The listing builds one solid part. Answer for the finished solid, in the listing's coordinates (mm). A direction names the side the tool comes from. Coordinates: 2 decimals unless noted, no trailing zeros. Write each loop counter-clockwise with the first axis right and the second up, starting at its lowest first coordinate (ties: lowest second). Pieces come first, ordered by that corner, then holes.
from build123d import *

# Parameters (mm, degrees)
BOSS_EXTRU_1_DEPTH        = 13
COQUE1_T                  = -5
COQUE1_THICKNESS_2_FACE_W = 65
COQUE1_THICKNESS_2_FACE_H = 65
COQUE1_THICKNESS_2_DEPTH  = 2
ENL_V_MAT_EXTRU_1_REACH   = 88.587
ESQUISSE2_R               = 2.5
ENL_V_MAT_EXTRU_2_REACH   = 95.396
ESQUISSE3_R               = 2.5
ESQUISSE4_W               = 18
ESQUISSE4_H               = 18
ESQUISSE4_W_2             = 15
ESQUISSE4_H_2             = 15
BOSS_EXTRU_2_DEPTH        = 10
ESQUISSE5_R               = 11.5
ESQUISSE5_R_2             = 14.5
ENL_V_MAT_EXTRU_3_DEPTH   = 13


with BuildPart() as part:
    # Esquisse1 → Boss.-Extru.1 (new body)
    with BuildSketch(Plane.XY):
        Polygon((44.118436308, 33.728448276), (54.118436308, 33.728448276), (54.118436308, 23.728448276), (54.118436308, -41.271551724), (-20.881563692, -41.271551724), (-20.881563692, 33.728448276), align=None)
    extrude(amount=BOSS_EXTRU_1_DEPTH)

    # Coque1
    coque1_openings = [part.faces().sort_by_distance(p)[0] for p in [
        (16.618436308, -3.771551724, 13),
    ]]
    offset(amount=COQUE1_T, openings=coque1_openings, kind=Kind.INTERSECTION)

    # Coque1 thickness 2 face (on inner face of the shell) → Coque1 thickness 2 (cut)
    with BuildSketch(Plane(origin=(16.618436308, -3.771551724, 5), x_dir=(-1, 0, 0), z_dir=(0, 0, -1))):
        Rectangle(COQUE1_THICKNESS_2_FACE_W, COQUE1_THICKNESS_2_FACE_H)
    extrude(amount=COQUE1_THICKNESS_2_DEPTH, mode=Mode.SUBTRACT)

    # Enlèv. mat.-Extru.1: up to this face of the body (flat: up to its plane)
    enl_v_mat_extru_1_end = Plane(part.part.faces().sort_by_distance((54.118436308, -3.771551724, 6.5))[0])
    # Esquisse2 → Enlèv. mat.-Extru.1 (cut, up to the picked face)
    with BuildSketch(Plane.ZY.offset(20.881563692), mode=Mode.PRIVATE) as enl_v_mat_extru_1_sk1:
        with Locations(Location((8, -16.271551724, 0), (0, 0, 270))):
            Circle(ESQUISSE2_R)
    enl_v_mat_extru_1_tool1 = split(extrude(enl_v_mat_extru_1_sk1.sketch, amount=-ENL_V_MAT_EXTRU_1_REACH, mode=Mode.PRIVATE), bisect_by=enl_v_mat_extru_1_end, keep=Keep.BOTH, mode=Mode.PRIVATE)
    # Esquisse2 → Enlèv. mat.-Extru.1 (cut, up to the picked face)
    with BuildSketch(Plane.ZY.offset(20.881563692), mode=Mode.PRIVATE) as enl_v_mat_extru_1_sk2:
        with Locations(Location((8, 8.728448276, 0), (0, 0, 270))):
            Circle(ESQUISSE2_R)
    enl_v_mat_extru_1_tool2 = split(extrude(enl_v_mat_extru_1_sk2.sketch, amount=-ENL_V_MAT_EXTRU_1_REACH, mode=Mode.PRIVATE), bisect_by=enl_v_mat_extru_1_end, keep=Keep.BOTH, mode=Mode.PRIVATE)
    add(enl_v_mat_extru_1_tool1.solids().sort_by(Axis((-20.881564, -16.271552, 8), (1, 0, 0)))[0], mode=Mode.SUBTRACT)
    add(enl_v_mat_extru_1_tool2.solids().sort_by(Axis((-20.881564, 8.728448, 8), (1, 0, 0)))[0], mode=Mode.SUBTRACT)

    # Enlèv. mat.-Extru.2: up to this face of the body (flat: up to its plane)
    enl_v_mat_extru_2_end = Plane(part.part.faces().sort_by_distance((16.618436308, 33.728448276, 6.5))[0])
    # Esquisse3 → Enlèv. mat.-Extru.2 (cut, up to the picked face)
    with BuildSketch(Plane.XZ.offset(41.271551724), mode=Mode.PRIVATE) as enl_v_mat_extru_2_sk1:
        with Locations(Location((4.118436308, 8, 0), (0, 0, 270))):
            Circle(ESQUISSE3_R)
    enl_v_mat_extru_2_tool1 = split(extrude(enl_v_mat_extru_2_sk1.sketch, amount=-ENL_V_MAT_EXTRU_2_REACH, mode=Mode.PRIVATE), bisect_by=enl_v_mat_extru_2_end, keep=Keep.BOTH, mode=Mode.PRIVATE)
    # Esquisse3 → Enlèv. mat.-Extru.2 (cut, up to the picked face)
    with BuildSketch(Plane.XZ.offset(41.271551724), mode=Mode.PRIVATE) as enl_v_mat_extru_2_sk2:
        with Locations(Location((29.118436308, 8, 0), (0, 0, 270))):
            Circle(ESQUISSE3_R)
    enl_v_mat_extru_2_tool2 = split(extrude(enl_v_mat_extru_2_sk2.sketch, amount=-ENL_V_MAT_EXTRU_2_REACH, mode=Mode.PRIVATE), bisect_by=enl_v_mat_extru_2_end, keep=Keep.BOTH, mode=Mode.PRIVATE)
    add(enl_v_mat_extru_2_tool1.solids().sort_by(Axis((4.118436, -41.271552, 8), (0, 1, 0)))[0], mode=Mode.SUBTRACT)
    add(enl_v_mat_extru_2_tool2.solids().sort_by(Axis((29.118436, -41.271552, 8), (0, 1, 0)))[0], mode=Mode.SUBTRACT)

    # Esquisse4 → Boss.-Extru.2 (add)
    with BuildSketch(Plane.XY.offset(3)):
        Polygon((-5.881563692, 28.728448276), (-15.881563692, 18.728448276), (-15.881563692, 28.728448276), align=None)
        Polygon((49.118436308, 28.728448276), (49.118436308, 18.728448276), (39.118436308, 28.728448276), align=None)
        with Locations((45.118436308, -32.271551724)):
            Rectangle(ESQUISSE4_W, ESQUISSE4_H)
        with Locations((-13.381563692, -33.771551724)):
            Rectangle(ESQUISSE4_W_2, ESQUISSE4_H_2)
    extrude(amount=BOSS_EXTRU_2_DEPTH)

    # Esquisse5 → Enlèv. mat.-Extru.3 (cut)
    with BuildSketch(Plane.XY.offset(13)):
        with Locations((-20.881563692, -41.271551724)):
            Circle(ESQUISSE5_R)
        with Locations((54.118436308, -41.271551724)):
            Circle(ESQUISSE5_R_2)
    extrude(amount=-ENL_V_MAT_EXTRU_3_DEPTH, mode=Mode.SUBTRACT)


solid = part.part
Q1. The part is cut by section B-B, the plane z = 8. State how many separate pieces and enclosed holes the cut face has, then the cut area to 3 significant figures.
Answers below:
separate pieces: 8
enclosed holes: 0
area: 1,300 mm2
Q2. The part is cut by section A-A, the plane y = -12.5. Write down the section's boundary in (x, z).
Answers below:
outline: (-20.88, 0) - (54.12, 0) - (54.12, 13) - (49.12, 13) - (49.12, 3) - (-15.88, 3) - (-15.88, 13) - (-20.88, 13) - close
Q3. Find the intervals of material crossed by probe 1 along X at (y, z) = (12.5, 4.5); probe 2 along Y at (x, z) = (34, 11.25); probe 3 along Y at (x, z) = (36.5, 6), in increasing order.
Answers below:
probe 1: x = -20.88 to -15.88, 49.12 to 54.12
probe 2: y = -41.27 to -36.27, 28.73 to 33.73
probe 3: y = -41.27 to -23.27, 28.73 to 33.73
Q4. The part is cut by section D-D, the plane z = 2. Write down the section's boundary in (x, y), then the cut area to 3 significant figures.
Answers below:
outline: (-20.88, -29.77) arc R11.5 cw to (-9.38, -41.27) - (39.62, -41.27) arc R14.5 cw to (54.12, -26.77) - (54.12, 33.73) - (-20.88, 33.73) - close
area: 5,360 mm2
Q5. Given pin 1 (3 mm diameter, centred on x = 34, y = -5.5, fed in from +Z); pin 2 (3 mm diameter, centred on y = -31, z = 6.5, fed in from +X); pin 3 (4 mm diameter, centred on x = 4.12, z = 8, fed in from -Y), each flat-ended and moving along its own axis, determine where each tip first touches the part or whether it passes through.
Answers below:
pin 1: stops at z = 3
pin 2: stops at x = 45.65
pin 3: passes through
Q6. Determine the mould class of faces 1 (the face through (-11, -26.272, 8)), 2 (the face through (17, 33.728, 6)), 3 (the face through (-12.66, -33.23, 6.59)), 4 (the face through (17, 30, 13)) for opening direction Y: released by +Y, released by -Y, zero draft, split by the parting line, or undercut.
Answers below:
face 1: undercut
face 2: released by +Y
face 3: released by -Y
face 4: zero draft
Q7. Which of the six approach directions +Z, -Z, +X, -X, +Y, -Y give full straight-line access (tool end or side, diameter ignored) to faces 5 (the face through (31.6, -38.8, 8.3)), 6 (the face through (17, 28.728, 8))?
Answers below:
face 5: +Y, -Y
face 6: +Z
Q8. The part is cut by section C-C, the plane x = -2. Write down the section's boundary in (y, z).
Answers below:
outline: (-41.27, 0) - (33.73, 0) - (33.73, 13) - (28.73, 13) - (28.73, 3) - (-36.27, 3) - (-36.27, 13) - (-41.27, 13) - close
